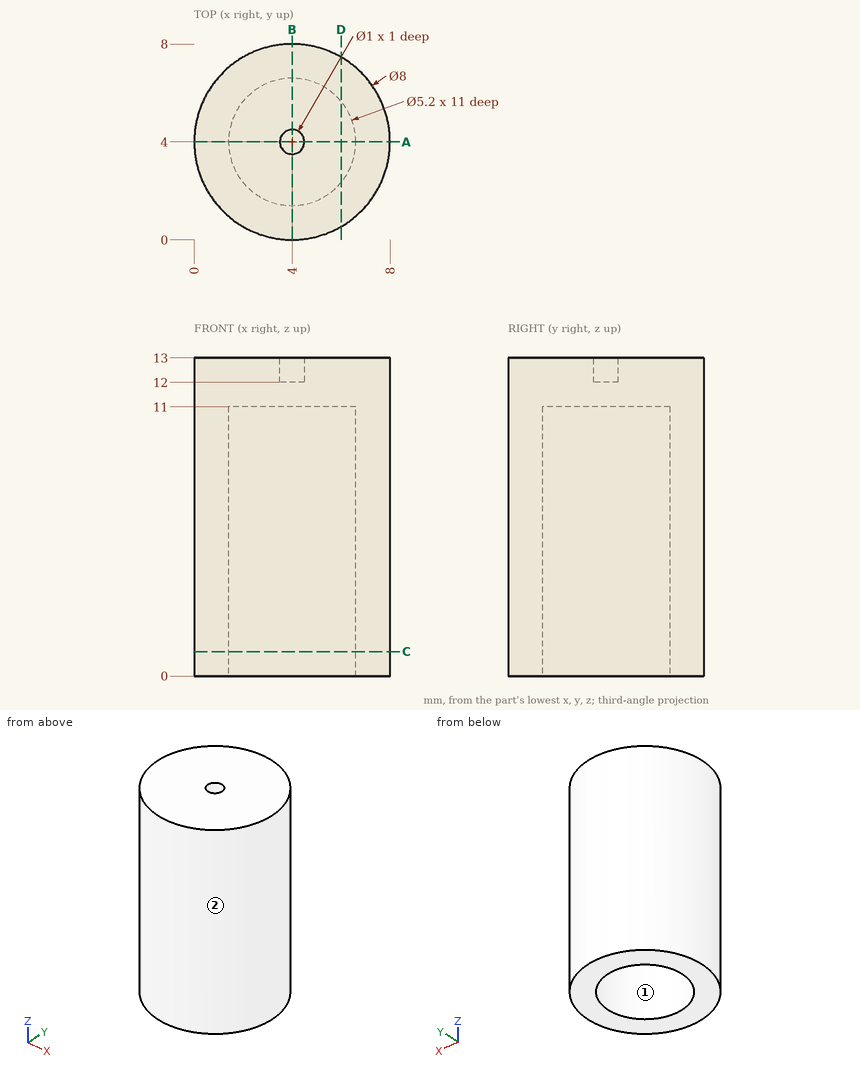
Geometry: see drawing. Coordinates: mm, zero at the bounding-box minimum. A direction names the side the tool comes from. Round coordinates to 2 decimals unless told otherwise and drop trailing zeros. Loops run counter-clockwise (first coordinate to the right, second up) from the corner with the lowest first, then second, coordinate; pieces in that order, holes last. Notation, with made-up numbers: M -34.75,-2.5 L -8.75,-2.5 A22 cw -8.75,22.5 Z; hole C 59,36.25 d4. An arc over 180 degrees is marked long. Use a Markdown table: item, result. Add a question column.
1. Contact query for flat-ended pins moving along their axis: pin 1 (4 mm diameter, centred on x = 1.5, z = 8.5, fed in from -Y); pin 2 (4 mm diameter, centred on x = 4, y = 4, fed in from -Z). Output: stop coordinate, or through.
2. Cut plane A-A, the plane y = 4. Output: boundary loops of the cut face in (x, z), and give its area (3 significant figures).
3. Set-up query: the marked faces 1 and 2. Return all of +Z, -Z, +X, -X, +Y, -Y with unobstructed straight access to the full face (end or side cutting, diameter ignored); none if empty.
4. Cut plane C-C, the plane z = 1. Output: boundary loops of the cut face in (x, y), and give its area (3 significant figures).
5. Ray query, line 1 along Y through (x, z) = (4, 12.55); line 2 along Y through (x, z) = (4, 7.75); line 3 along Z through (x, y) = (4.5, 1.75). Return the intervals inside material, ascending. Write a range as [from, to].
6. Cut plane D-D, the plane x = 6. Output: boundary loops of the cut face in (y, z).
Solution:
| question | item | result |
|---|---|---|
| 1 | pin 1 | stops at y = 0.03 |
| 1 | pin 2 | stops at z = 11 |
| 2 | outline | M 0,0 L 1.4,0 L 1.4,11 L 6.6,11 L 6.6,0 L 8,0 L 8,13 L 4.5,13 L 4.5,12 L 3.5,12 L 3.5,13 L 0,13 Z |
| 2 | area | 45.8 mm2 |
| 3 | face 1 | -Z |
| 3 | face 2 | +Z, -Z |
| 4 | outline | C 4,4 d8; hole C 4,4 d5.2 |
| 4 | area | 29.0 mm2 |
| 5 | line 1 | y = [0, 3.5], [4.5, 8] |
| 5 | line 2 | y = [0, 1.4], [6.6, 8] |
| 5 | line 3 | z = [11, 13] |
| 6 | outline | M 0.54,0 L 2.34,0 L 2.34,11 L 5.66,11 L 5.66,0 L 7.46,0 L 7.46,13 L 0.54,13 Z |
